```python
from build123d import *

# Parameters (mm, degrees)
SKIZZE1_R                       = 8.5
AUFSATZ_LINEAR_AUSTRAGEN1_DEPTH = 33.5
SKIZZE2_R                       = 3.799988553
AUFSATZ_LINEAR_AUSTRAGEN2_DEPTH = 1
VERRUNDUNG1_R                   = 1.5
VERRUNDUNG2_R                   = 0.5
SKIZZE3_R                       = 5
SKIZZE3_R_2                     = 3.799988553
SCHNITT_LINEAR_AUSTRAGEN1_DEPTH = 0.005


with BuildPart() as part:
    # Skizze1 → Aufsatz-Linear austragen1 (new body)
    with BuildSketch(Plane(origin=(0, 0, 0), x_dir=(1, 0, 0), z_dir=(0, 1, 0))):
        Circle(SKIZZE1_R)
    extrude(amount=AUFSATZ_LINEAR_AUSTRAGEN1_DEPTH)

    # Skizze2 → Aufsatz-Linear austragen2 (add)
    with BuildSketch(Plane(origin=(0, 33.5, 0), x_dir=(1, 0, 0), z_dir=(0, 1, 0))):
        Circle(SKIZZE2_R)
    extrude(amount=AUFSATZ_LINEAR_AUSTRAGEN2_DEPTH)

    # Verrundung1
    verrundung1_edges = [part.edges().sort_by_distance(p)[0] for p in [
        (-8.5, 0, 0),
        (-8.5, 33.5, 0),
    ]]
    fillet(verrundung1_edges, radius=VERRUNDUNG1_R)

    # Verrundung2
    verrundung2_edges = [part.edges().sort_by_distance(p)[0] for p in [
        (-3.799988553, 34.5, 0),
    ]]
    fillet(verrundung2_edges, radius=VERRUNDUNG2_R)

    # Skizze3 → Schnitt-Linear austragen1 (cut)
    with BuildSketch(Plane(origin=(0, 33.5, 0), x_dir=(1, 0, 0), z_dir=(0, 1, 0))):
        Circle(SKIZZE3_R)
        Circle(SKIZZE3_R_2, mode=Mode.SUBTRACT)
    extrude(amount=-SCHNITT_LINEAR_AUSTRAGEN1_DEPTH, mode=Mode.SUBTRACT)


solid = part.part
```
The listing builds one solid part. Answer for the finished solid, in the listing's coordinates (mm). A direction names the side the tool comes from. Coordinates: 2 decimals unless noted, no trailing zeros. Write each loop counter-clockwise with the first axis right and the second up, starting at its lowest first coordinate (ties: lowest second). Pieces come first, ordered by that corner, then holes. Notation, with made-up numbers: (80.25, 76.5) - (103.25, 76.5) arc R14 cw to (103.25, 85.5) - close; hole circle Ø11 at (76, 81). An arc over 180 degrees is marked (long way). Return JSON: item names as keys, results as strings. Group by question number.
Q1. Flat-ended cylindrical pins translate along their axes: pin 1 Ø4 at (x, y) = (3, 14) entering from -Z; pin 2 Ø8 at (y, z) = (24.5, -6) entering from -X; pin 3 Ø10 at (x, y) = (5.5, 12) entering from +Z. Find the tip coordinate at first contact, or state that the pin passes through.
Q2. The part is cut by section A-A on z = 0. Write down the section's boundary in (x, y) (3 decimals).
Q3. The part is cut by section B-B on x = 0. Write down the section's boundary in (y, z) (3 decimals), and give its area (3 significant figures).
Q4. Find the intervals of material crossed by line 1 along Y through (x, z) = (-3.25, -4); line 2 along Y through (x, z) = (6.75, 5); line 3 along X through (y, z) = (28, 7.5), in increasing order. Write a range as [from, to].
Q5. The part is cut by section C-C on y = 18. Write down the section's boundary in (x, z), and give its area (3 significant figures).
Q6. Which of the six approach directions +Z, -Z, +X, -X, +Y, -Y give full straight-line access (tool end or side, diameter ignored) to faces 1 (the flat face through (-2, 33.5, -5)), 2 (the cylindrical face through (4.57, 16.536, -7.167))?
Evaluation:
{
 "1": {"pin 1": "stops at z = -8.44", "pin 2": "stops at x = -8.26", "pin 3": "stops at z = 8.49"},
 "2": {"outline": "(-8.5, 1.5) arc R1.5 ccw to (-7, 0) - (7, 0) arc R1.5 ccw to (8.5, 1.5) - (8.5, 32) arc R1.5 ccw to (7, 33.5) - (5, 33.5) - (5, 33.495) - (3.8, 33.495) - (3.8, 34) arc R0.5 ccw to (3.3, 34.5) - (-3.3, 34.5) arc R0.5 ccw to (-3.8, 34) - (-3.8, 33.495) - (-5, 33.495) - (-5, 33.5) - (-7, 33.5) arc R1.5 ccw to (-8.5, 32) - close"},
 "3": {"outline": "(0, -7) arc R1.5 ccw to (1.5, -8.5) - (32, -8.5) arc R1.5 ccw to (33.5, -7) - (33.5, -5) - (33.495, -5) - (33.495, -3.8) - (34, -3.8) arc R0.5 ccw to (34.5, -3.3) - (34.5, 3.3) arc R0.5 ccw to (34, 3.8) - (33.495, 3.8) - (33.495, 5) - (33.5, 5) - (33.5, 7) arc R1.5 ccw to (32, 8.5) - (1.5, 8.5) arc R1.5 ccw to (0, 7) - close", "area": "575 mm2"},
 "4": {"line 1": "y = [0, 33.5]", "line 2": "y = [0.96, 32.54]", "line 3": "x = [-4, 4]"},
 "5": {"outline": "circle Ø17 at (0, 0)", "area": "227 mm2"},
 "6": {"face 1": "+Y", "face 2": "+Y, -Y"}
}
